from build123d import *

# Parameters (mm, degrees)
SKETCH2_R           = 1.57
BOSS_EXTRUDE1_DEPTH = 5
SKETCH3_R           = 1.57
CUT_EXTRUDE1_DEPTH  = 8


with BuildPart() as part:
    # Sketch2 → Boss-Extrude1 (new body)
    with BuildSketch(Plane(origin=(0, 0, 0), x_dir=(1, 0, 0), z_dir=(0, 1, 0))):
        Polygon((-5, 1.830127019), (-5, 0), (-5, -14), (5, -14), (5, 0), (5, 1.830127019), (2.5, 4.330127019), (-2.5, 4.330127019), align=None)
        Circle(SKETCH2_R, mode=Mode.SUBTRACT)
    extrude(amount=BOSS_EXTRUDE1_DEPTH)

    # Sketch3 → Cut-Extrude1 (cut)
    with BuildSketch(Plane.XY.offset(14)):
        with Locations((0, 2.5)):
            Circle(SKETCH3_R)
    extrude(amount=-CUT_EXTRUDE1_DEPTH, mode=Mode.SUBTRACT)


solid = part.part
Input: part model. Units: mm. Frame: model coordinates. A direction names the side the tool comes from. Coordinates: 2 decimals unless noted, no trailing zeros. Loops run counter-clockwise (first coordinate to the right, second up) from the corner with the lowest first, then second, coordinate; pieces in that order, holes last. Notation, with made-up numbers: (-39.5, 63) -> (8.5, 63) arc R24 ccw to (8.5, 83) -> close; hole circle Ø8 at (84.25, 52). An arc over 180 degrees is marked (long way). Write each question's results on one line, items separated by ' | '. Start each with the question number.
Q1. Reachability of faces 4 (the cylindrical face through (0.724, 1.107, 10.056)), 5 (the cylindrical face through (1.5, 2.46, -0.47)) from +Z, -Z, +X, -X, +Y, -Y: full face, straight path, thin tool, end or side. Return the list, or none.
Q2. Ray query, line 1 (X direction, y = 2, z = 0); line 2 (Y direction, x = 0, z = 10.25); line 3 (Z direction, x = 0.25, y = 2.75). Return the intervals inside material, ascending. Write a range as from..to.
Q3. Pull-direction query (X, two-part tool) for faces 1 (the flat face through (5, 2, 6)), 2 (the flat face through (0, 3, 6)), 3 (the flat face through (0, 0, 5)); classes: released by +X, released by -X, zero draft, split by the parting line, or undercut.
Q4. Section B-B, the plane x = 0. Return the cut outline in (y, z), plus the area to 3 significant figures.
Q5. Section A-A, the plane z = 0. Return the cut outline in (x, y), plus the area to 3 significant figures.
Q6. Section D-D, the plane z = 13. Return the cut outline in (x, y).
Q7. Section C-C, the plane y = 0.65. Return the cut outline in (x, z).
Found:
1) face 4: +Z | face 5: +Y, -Y
2) line 1: -5..-1.57, 1.57..5 | line 2: 0..0.93, 4.07..5 | line 3: -4.33..-1.55, 1.55..6
3) face 1: released by +X | face 2: undercut | face 3: zero draft
4) outline: (0, -4.33) -> (5, -4.33) -> (5, -1.57) -> (0, -1.57) -> close; (0, 1.57) -> (5, 1.57) -> (5, 14) -> (4.07, 14) -> (4.07, 6) -> (0.93, 6) -> (0.93, 14) -> (0, 14) -> close | area: 50.8 mm2
5) outline: (-5, 0) -> (-1.57, 0) -> (-1.57, 5) -> (-5, 5) -> close; (1.57, 0) -> (5, 0) -> (5, 5) -> (1.57, 5) -> close | area: 34.3 mm2
6) outline: (-5, 0) -> (5, 0) -> (5, 5) -> (-5, 5) -> close; hole circle Ø3.14 at (0, 2.5)
7) outline: (-5, -1.83) -> (-2.5, -4.33) -> (2.5, -4.33) -> (5, -1.83) -> (5, 14) -> (-5, 14) -> close; hole circle Ø3.14 at (0, 0)
